The drawing under review shows one solid part. Ordinate dimensions are in mm from its lowest x, y, z. Give positions to 0.01 mm unless a question says otherwise; leave off trailing zeros. Write each loop counter-clockwise with the first axis right and the second up, starting at its lowest first coordinate (ties: lowest second). Pieces come first, ordered by that corner, then holes. Notation, with made-up numbers: M 49.5,9.25 L 87.5,9.25 A18 cw 87.5,33.25 Z; hole C -36,29.25 d11. An arc over 180 degrees is marked long. Write each question's results on one line, items separated by ' | '. Start each with the question number.
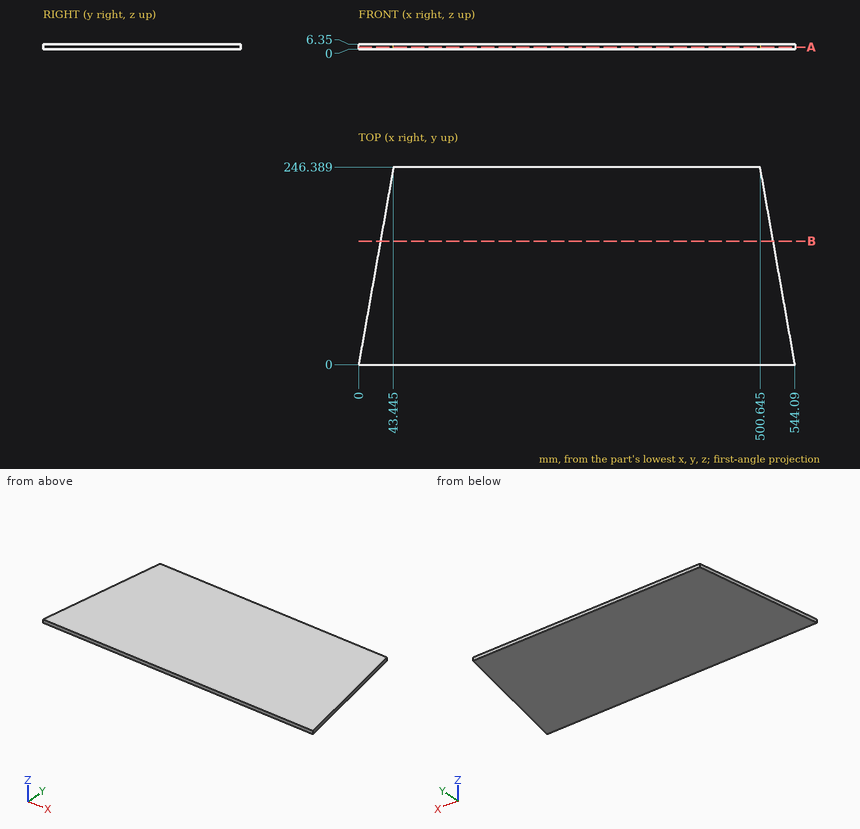
Q1. For pin 1 Ø3 at (y, z) = (209, 3) entering from +X, flat-tipped, find the tip position at first contact; note if it passes through.
Q2. We need section B-B on y = 154. Write out the cut boundary in (x, z), and give its area (3 significant figures).
Q3. We need section A-A on z = 2.5. Write out the cut boundary in (x, y) (3 decimals).
Q4. Wall thickness on line 1 along X through (y, z) = (84.5, 1.75); line 2 along X through (y, z) = (104.5, 1.75): over which ranges is each line inside the solid? List them lowest first. Write a range as from..to.
Answer sheet:
1) pin 1: x = 507.5
2) outline: M 27.15,0 L 516.94,0 L 516.94,6.35 L 27.15,6.35 Z | area: 3,110 mm^2
3) outline: M 0,0 L 544.09,0 L 500.645,246.389 L 43.445,246.389 Z
4) line 1: 14.9..529.19 | line 2: 18.43..525.66
